```python
from build123d import *

# Parameters (mm, degrees)
F0_W      = 101.6
F0_H      = 152.4
F1_DEPTH  = 19.05
F3_D      = 6.5278
F2_R      = 23.8125
F4_DEPTH  = 19.051
F6_DEPTH  = 19.051
F7_W      = 101.6
F7_H      = 25.4
F8_DEPTH  = 19.051
F10_D     = 6.3754
F10_DEPTH = 16.9418
F10_TIP   = 1.9153633953
F11_D     = 6.5278
F11_DEPTH = 28.3633333333
F11_TIP   = 1.9611489744


with BuildPart() as f1:
    # F0 (on Top) → F1 (new body)
    with BuildSketch(Plane.XY):
        with Locations((0, 12.7)):
            Rectangle(F0_W, F0_H)
    extrude(amount=F1_DEPTH)

    # F3 (through all)
    with Locations(Plane.XY.offset(19.05)):
        with Locations((-29.9042528832, 55.3042528832), (29.9042528832, 55.3042528832), (29.9042528832, -4.5042528832), (-29.9042528832, -4.5042528832)):
            Hole(F3_D / 2)

    # F2 (on face) → F4 (cut, through all)
    with BuildSketch(Plane.XY.offset(19.05)):
        with Locations((0, 25.4)):
            Circle(F2_R)
    extrude(amount=-F4_DEPTH, mode=Mode.SUBTRACT)

    # F5 (on face) → F6 (cut, through all)
    with BuildSketch(Plane.XY.offset(19.05)):
        with BuildLine():
            Line((-23.8106845457, 88.9), (-23.8106845457, 25.6940369276))
            ThreePointArc((-23.8106845457, 25.6940369276), (-17.0245539834, 8.5843833211), (0, 1.5875))
            ThreePointArc((0, 1.5875), (16.8536210319, 8.7422088532), (23.81087373, 25.6782956372))
            Line((23.81087373, 25.6782956372), (23.81087373, 88.9))
            Line((23.81087373, 88.9), (-23.8106845457, 88.9))
        make_face()
    extrude(amount=-F6_DEPTH, mode=Mode.SUBTRACT)

    # F7 (on face) → F8 (cut, through all)
    with BuildSketch(Plane.XY.offset(19.05)):
        with Locations((0, 76.2)):
            Rectangle(F7_W, F7_H)
    extrude(amount=-F8_DEPTH, mode=Mode.SUBTRACT)

    # F10
    with Locations(Plane.XZ.offset(63.5)):
        with Locations((-38.1, 9.525), (38.1, 9.525)):
            Hole(F10_D / 2, depth=F10_DEPTH)
            with Locations((0, 0, -(F10_DEPTH + F10_TIP / 2))):  # 118° drill point
                Cone(0, F10_D / 2, F10_TIP, mode=Mode.SUBTRACT)

    # F11
    with Locations(Plane.XZ.offset(63.5)):
        with Locations((-22.225, 9.525), (22.225, 9.525)):
            Hole(F11_D / 2, depth=F11_DEPTH)
            with Locations((0, 0, -(F11_DEPTH + F11_TIP / 2))):  # 118° drill point
                Cone(0, F11_D / 2, F11_TIP, mode=Mode.SUBTRACT)


solid = f1.part
```
Source: CAD feature listing. Evaluate the final solid. Frame: model axes, mm. A direction names the side the tool comes from. Coordinates: 2 decimals unless noted, no trailing zeros. Write each loop counter-clockwise with the first axis right and the second up, starting at its lowest first coordinate (ties: lowest second). Pieces come first, ordered by that corner, then holes. Notation, with made-up numbers: (-36, 53) - (19, 53) arc R25 ccw to (19, 79) - close; hole circle Ø4 at (41.25, 31). An arc over 180 degrees is marked (long way). Answer as a JSON object with one key per item and string values.
Q1. Section query C-C, the plane y = -40. Output: boundary loops of the cut face in (x, z) (3 decimals), plus the area to 3 significant figures.
Ans:
{"outline": "(-50.8, 0) - (50.8, 0) - (50.8, 19.05) - (-50.8, 19.05) - close; hole circle Ø6.528 at (-22.225, 9.525); hole circle Ø6.528 at (22.225, 9.525)", "area": "1,870 mm2"}
Q2. First-contact query: pin 1 Ø6 at (x, z) = (-22.225, 9.525) entering from +Y; pin 2 Ø8 at (x, z) = (-15, 10) entering from +Y; pin 3 Ø5.5 at (x, z) = (-38.1, 9.525) entering from -Y. Flat tips, straight axial feed; report the tip coordinate or a pass-through.
Ans:
{"pin 1": "stops at y = 63.5", "pin 2": "stops at y = 10.86", "pin 3": "stops at y = -46.3"}
Q3. Section query D-D, the plane x = -6.5. Output: boundary loops of the cut face in (y, z).
Ans:
{"outline": "(-63.5, 0) - (2.42, 0) - (2.42, 19.05) - (-63.5, 19.05) - close"}
Q4. Draft query along Z for faces 4 (the flat face through (-37, 63.5, 10)), 5 (the cylindrical face through (19.2, -49.1, 8.3)), 6 (the flat face through (-1, -13, 19.05)), 7 (the cylindrical face through (40.45, -54.91, 11.68)). Return one class per face: released by +Z, released by -Z, zero draft, split by the parting line, or undercut.
Ans:
{"face 4": "zero draft", "face 5": "undercut", "face 6": "released by +Z", "face 7": "undercut"}
Q5. Section query B-B, the plane x = 31. Output: boundary loops of the cut face in (y, z).
Ans:
{"outline": "(-63.5, 0) - (-7.58, 0) - (-7.58, 19.05) - (-63.5, 19.05) - close; (-1.43, 0) - (52.23, 0) - (52.23, 19.05) - (-1.43, 19.05) - close; (58.38, 0) - (63.5, 0) - (63.5, 19.05) - (58.38, 19.05) - close"}
Q6. Section query A-A, the plane y = 40. Output: boundary loops of the cut face in (x, z).
Ans:
{"outline": "(-50.8, 0) - (-23.81, 0) - (-23.81, 19.05) - (-50.8, 19.05) - close; (23.81, 0) - (50.8, 0) - (50.8, 19.05) - (23.81, 19.05) - close"}
Q7. Set-up query: faces 1 (the flat face through (37, 63.5, 10)), 2 (the flat face through (-23.811, 45, 10)), 3 (the cylindrical face through (-41.14, -54.91, 10.48)). Return all of +Z, -Z, +X, -X, +Y, -Y with unobstructed straight access to the full face (end or side cutting, diameter ignored); none if empty.
Ans:
{"face 1": "+Z, -Z, +X, -X, +Y", "face 2": "+Z, -Z, +Y", "face 3": "-Y"}
Q8. Material intervals for line 1 (Y direction, x = 28, z = 8.25); line 2 (X direction, y = 39.5, z = 14.75); line 3 (X direction, y = -5.5, z = 4.5), sorted ascending. Write a range as [from, to].
Ans:
{"line 1": "y = [-63.5, -7.16], [-1.85, 52.65], [57.96, 63.5]", "line 2": "x = [-50.8, -23.81], [23.81, 50.8]", "line 3": "x = [-50.8, -33.01], [-26.8, 26.8], [33.01, 50.8]"}
